from build123d import *

# Parameters (mm, degrees)
SKETCH1_R           = 1.517913389
SKETCH1_R_2         = 1.5
BOSS_EXTRUDE1_DEPTH = 5.08


with BuildPart() as part:
    # Sketch1 → Boss-Extrude1 (new body)
    with BuildSketch(Plane(origin=(0, 0, 0), x_dir=(-1, 0, 0), z_dir=(0, 0, 1))):
        with BuildLine():
            ThreePointArc((109.76359006, -85.328738191), (97.326662127, -86.828738191), (109.76359006, -88.328738191))
            Line((109.76359006, -88.328738191), (110.405158411, -88.328738191))
            Line((110.405158411, -88.328738191), (113.735498826, -88.328738191))
            Line((113.735498826, -88.328738191), (117.281412131, -88.328738191))
            Line((117.281412131, -88.328738191), (117.281412131, -101.902374013))
            ThreePointArc((117.281412131, -101.902374013), (114.305617027, -109.08657891), (107.121412131, -112.062374013))
            Line((107.121412131, -112.062374013), (94.361674585, -112.062374013))
            Line((94.361674585, -112.062374013), (94.361674585, -111.794978321))
            Line((94.361674585, -111.794978321), (94.361674585, -64.328592097))
            Line((94.361674585, -64.328592097), (117.281412131, -64.328592097))
            Line((117.281412131, -64.328592097), (117.281412131, -85.328738191))
            Line((117.281412131, -85.328738191), (113.735498826, -85.328738191))
            Line((113.735498826, -85.328738191), (110.405158411, -85.328738191))
            Line((110.405158411, -85.328738191), (109.76359006, -85.328738191))
        make_face()
        with Locations(Location((103.635582515, -69.140487693, 0), (0, 0, 180))):
            Circle(SKETCH1_R, mode=Mode.SUBTRACT)
        with Locations(Location((103.635582515, -104.844491412, 0), (0, 0, 180))):
            Circle(SKETCH1_R_2, mode=Mode.SUBTRACT)
    extrude(amount=BOSS_EXTRUDE1_DEPTH)


solid = part.part
Model file for the job. Use its own axes, mm. A direction names the side the tool comes from. Round coordinates to 2 decimals unless told otherwise and drop trailing zeros. Order: outer loops, then holes, each group sorted by start corner. A loop starts at its lowest first (then second) coordinate and runs counter-clockwise, first axis right, second up.
(1) Band-saw the part on C-C (x = -109). List the corners of the cut face in (y, z).
(2) 3-axis set-ups, long thin cutter, end or side, ignore diameter. For faces 1 (the face through (-114.38, 109.01, 2.5)), 2 (the face through (-114, 85.329, 3)): which of +Z, -Z, +X, -X, +Y, -Y reach the whole face in a straight line?
(3) Band-saw the part on A-A (x = -106). List the corners of the cut face in (y, z), then the cut area to 3 significant figures.
(4) Pull direction X, two halves, no side cores. Call faces 3 (the face through (-113, 88.329, 3)), 4 (the face through (-117.281, 95, 3)), 5 (the face through (-97.33, 86.57, 2.5)): released by +X, released by -X, zero draft, split by the parting line, or undercut.
(5) Drill centre lines: line 1 (Y direction, x = -105, z = 1.1); line 2 (Y direction, x = -104.25, z = 3.9); line 3 (X direction, y = 90, z = 0.85). Where is each one in solid material? Low to high.
(6) Pin check, flat tip, straight feed: pin 1 (1.5 mm diameter, centred on x = -114.5, z = 2, fed in from +Y). Stop position of the tip, or through.
(7) Band-saw the part on B-B (z = 1.45). List the corners of the cut face in (x, y).
Verdict:
1. outline: (64.33, 0) - (83.51, 0) - (83.51, 5.08) - (64.33, 5.08) - close; (90.15, 0) - (111.89, 0) - (111.89, 5.08) - (90.15, 5.08) - close
2. face 1: +Z, -Z, -X, +Y
2. face 2: +Z, -Z, -X
3. outline: (64.33, 0) - (80.98, 0) - (80.98, 5.08) - (64.33, 5.08) - close; (92.68, 0) - (112.06, 0) - (112.06, 5.08) - (92.68, 5.08) - close
3. area: 183 mm2
4. face 3: zero draft
4. face 4: released by -X
4. face 5: undercut
5. line 1: y = 64.33 to 68.48, 69.81 to 80.67, 92.99 to 104.22, 105.47 to 112.06
5. line 2: y = 64.33 to 67.75, 70.53 to 80.55, 93.11 to 103.48, 106.21 to 112.06
5. line 3: x = -117.28 to -109.09, -98.18 to -94.36
6. pin 1: stops at y = 109.6
7. outline: (-117.28, 64.33) - (-94.36, 64.33) - (-94.36, 112.06) - (-107.12, 112.06) arc R10.16 ccw to (-117.28, 101.9) - (-117.28, 88.33) - (-109.76, 88.33) arc R6.31 cw (long way) to (-109.76, 85.33) - (-117.28, 85.33) - close; hole circle Ø3.04 at (-103.64, 69.14); hole circle Ø3 at (-103.64, 104.84)
